from build123d import *

# Parameters (mm, degrees)
CYLINDER050_R           = 1.25
CYLINDER050_DEPTH       = 10
CYLINDER050_PITCH_ANGLE = 90
CYLINDER045_R           = 1.25
CYLINDER045_DEPTH       = 10
CYLINDER045_PITCH_ANGLE = 90
CYLINDER046_R           = 1.25
CYLINDER046_DEPTH       = 10
CYLINDER046_PITCH_ANGLE = 90
CYLINDER032_R           = 8.1
CYLINDER032_DEPTH       = 5
CYLINDER032_PITCH_ANGLE = 90
CYLINDER017_R           = 1.6
CYLINDER017_DEPTH       = 25
CYLINDER017_PITCH_ANGLE = 90
CYLINDER018_R           = 3.1
CYLINDER018_DEPTH       = 4
CYLINDER018_PITCH_ANGLE = 90
CYLINDER019_R           = 1.6
CYLINDER019_DEPTH       = 25
CYLINDER019_PITCH_ANGLE = 90
CYLINDER020_R           = 3.1
CYLINDER020_DEPTH       = 4
CYLINDER020_PITCH_ANGLE = 90
CYLINDER015_R           = 1.6
CYLINDER015_DEPTH       = 25
CYLINDER015_PITCH_ANGLE = 90
CYLINDER016_R           = 3.1
CYLINDER016_DEPTH       = 4
CYLINDER016_PITCH_ANGLE = 90
CYLINDER013_R           = 1.6
CYLINDER013_DEPTH       = 25
CYLINDER013_PITCH_ANGLE = 90
CYLINDER014_R           = 3.1
CYLINDER014_DEPTH       = 4
CYLINDER014_PITCH_ANGLE = 90
CYLINDER012_R           = 15.5
CYLINDER012_DEPTH       = 18
CYLINDER012_PITCH_ANGLE = 90
CYLINDER022_R           = 4
CYLINDER022_DEPTH       = 5
CYLINDER022_PITCH_ANGLE = 90
CYLINDER021_R           = 4
CYLINDER021_DEPTH       = 5
CYLINDER021_PITCH_ANGLE = 90
BOX007_W                = 33
BOX007_H                = 30
BOX007_DEPTH            = 40
CYLINDER003_R           = 17
CYLINDER003_DEPTH       = 19
CYLINDER003_PITCH_ANGLE = 90
BOX001_W                = 23
BOX001_H                = 30
BOX001_DEPTH            = 35
FILLET002_R             = 10
FILLET004_R             = 6
BOX_W                   = 32
BOX_H                   = 30
BOX_DEPTH               = 40
FILLET003_R             = 10
FILLET005_R             = 6


with BuildPart() as cylinder050:
    # Cylinder050 → Cylinder050 (new body)
    with BuildSketch(Plane.XY):
        Circle(CYLINDER050_R)
    extrude(amount=CYLINDER050_DEPTH)


with BuildPart() as cylinder050_1:
    # Cylinder050 pitch: moved
    add(cylinder050.part.rotate(Axis((0, 0, 0), (0, 1, 0)), CYLINDER050_PITCH_ANGLE))


with BuildPart() as cylinder050_2:
    # Cylinder050 placement: moved
    add(cylinder050_1.part.moved(Location((48, 15, 30))))


with BuildPart() as cylinder045:
    # Cylinder045 → Cylinder045 (new body)
    with BuildSketch(Plane.XY):
        Circle(CYLINDER045_R)
    extrude(amount=CYLINDER045_DEPTH)


with BuildPart() as cylinder045_1:
    # Cylinder045 pitch: moved
    add(cylinder045.part.rotate(Axis((0, 0, 0), (0, 1, 0)), CYLINDER045_PITCH_ANGLE))


with BuildPart() as cylinder045_2:
    # Cylinder045 placement: moved
    add(cylinder045_1.part.moved(Location((47, 7, 12))))


with BuildPart() as fusion023:
    # Cylinder046 → Cylinder046 (new body)
    with BuildSketch(Plane.XY):
        Circle(CYLINDER046_R)
    extrude(amount=CYLINDER046_DEPTH)


with BuildPart() as fusion023_1:
    # Cylinder046 pitch: moved
    add(fusion023.part.rotate(Axis((0, 0, 0), (0, 1, 0)), CYLINDER046_PITCH_ANGLE))


with BuildPart() as fusion023_2:
    # Cylinder046 placement: moved
    add(fusion023_1.part.moved(Location((46, 23, 12))))

    # Fusion023: union Cylinder045
    add(cylinder045_2.part)


with BuildPart() as cylinder032:
    # Cylinder032 → Cylinder032 (new body)
    with BuildSketch(Plane.XY):
        Circle(CYLINDER032_R)
    extrude(amount=CYLINDER032_DEPTH)


with BuildPart() as cylinder032_1:
    # Cylinder032 pitch: moved
    add(cylinder032.part.rotate(Axis((0, 0, 0), (0, 1, 0)), CYLINDER032_PITCH_ANGLE))


with BuildPart() as cylinder032_2:
    # Cylinder032 placement: moved
    add(cylinder032_1.part.moved(Location((51, 15, 19))))


with BuildPart() as cylinder017:
    # Cylinder017 → Cylinder017 (new body)
    with BuildSketch(Plane.XY):
        Circle(CYLINDER017_R)
    extrude(amount=CYLINDER017_DEPTH)


with BuildPart() as cylinder017_1:
    # Cylinder017 pitch: moved
    add(cylinder017.part.rotate(Axis((0, 0, 0), (0, 1, 0)), CYLINDER017_PITCH_ANGLE))


with BuildPart() as cylinder017_2:
    # Cylinder017 placement: moved
    add(cylinder017_1.part.moved(Location((30, 0, 19))))


with BuildPart() as fusion010:
    # Cylinder018 → Cylinder018 (new body)
    with BuildSketch(Plane.XY):
        Circle(CYLINDER018_R)
    extrude(amount=CYLINDER018_DEPTH)


with BuildPart() as fusion010_1:
    # Cylinder018 pitch: moved
    add(fusion010.part.rotate(Axis((0, 0, 0), (0, 1, 0)), CYLINDER018_PITCH_ANGLE))


with BuildPart() as fusion010_2:
    # Cylinder018 placement: moved
    add(fusion010_1.part.moved(Location((51, 0, 19))))

    # Fusion010: union Cylinder017
    add(cylinder017_2.part)


with BuildPart() as fusion010_3:
    # Fusion010 placement: moved
    add(fusion010_2.part.moved(Location((0, 25, 17))))


with BuildPart() as cylinder019:
    # Cylinder019 → Cylinder019 (new body)
    with BuildSketch(Plane.XY):
        Circle(CYLINDER019_R)
    extrude(amount=CYLINDER019_DEPTH)


with BuildPart() as cylinder019_1:
    # Cylinder019 pitch: moved
    add(cylinder019.part.rotate(Axis((0, 0, 0), (0, 1, 0)), CYLINDER019_PITCH_ANGLE))


with BuildPart() as cylinder019_2:
    # Cylinder019 placement: moved
    add(cylinder019_1.part.moved(Location((30, 0, 19))))


with BuildPart() as fusion011:
    # Cylinder020 → Cylinder020 (new body)
    with BuildSketch(Plane.XY):
        Circle(CYLINDER020_R)
    extrude(amount=CYLINDER020_DEPTH)


with BuildPart() as fusion011_1:
    # Cylinder020 pitch: moved
    add(fusion011.part.rotate(Axis((0, 0, 0), (0, 1, 0)), CYLINDER020_PITCH_ANGLE))


with BuildPart() as fusion011_2:
    # Cylinder020 placement: moved
    add(fusion011_1.part.moved(Location((51, 0, 19))))

    # Fusion011: union Cylinder019
    add(cylinder019_2.part)


with BuildPart() as fusion011_3:
    # Fusion011 placement: moved
    add(fusion011_2.part.moved(Location((0, 26, -14))))


with BuildPart() as cylinder015:
    # Cylinder015 → Cylinder015 (new body)
    with BuildSketch(Plane.XY):
        Circle(CYLINDER015_R)
    extrude(amount=CYLINDER015_DEPTH)


with BuildPart() as cylinder015_1:
    # Cylinder015 pitch: moved
    add(cylinder015.part.rotate(Axis((0, 0, 0), (0, 1, 0)), CYLINDER015_PITCH_ANGLE))


with BuildPart() as cylinder015_2:
    # Cylinder015 placement: moved
    add(cylinder015_1.part.moved(Location((30, 0, 19))))


with BuildPart() as fusion009:
    # Cylinder016 → Cylinder016 (new body)
    with BuildSketch(Plane.XY):
        Circle(CYLINDER016_R)
    extrude(amount=CYLINDER016_DEPTH)


with BuildPart() as fusion009_1:
    # Cylinder016 pitch: moved
    add(fusion009.part.rotate(Axis((0, 0, 0), (0, 1, 0)), CYLINDER016_PITCH_ANGLE))


with BuildPart() as fusion009_2:
    # Cylinder016 placement: moved
    add(fusion009_1.part.moved(Location((51, 0, 19))))

    # Fusion009: union Cylinder015
    add(cylinder015_2.part)


with BuildPart() as fusion009_3:
    # Fusion009 placement: moved
    add(fusion009_2.part.moved(Location((0, 5, 17))))


with BuildPart() as cylinder013:
    # Cylinder013 → Cylinder013 (new body)
    with BuildSketch(Plane.XY):
        Circle(CYLINDER013_R)
    extrude(amount=CYLINDER013_DEPTH)


with BuildPart() as cylinder013_1:
    # Cylinder013 pitch: moved
    add(cylinder013.part.rotate(Axis((0, 0, 0), (0, 1, 0)), CYLINDER013_PITCH_ANGLE))


with BuildPart() as cylinder013_2:
    # Cylinder013 placement: moved
    add(cylinder013_1.part.moved(Location((30, 0, 19))))


with BuildPart() as fusion013:
    # Cylinder014 → Cylinder014 (new body)
    with BuildSketch(Plane.XY):
        Circle(CYLINDER014_R)
    extrude(amount=CYLINDER014_DEPTH)


with BuildPart() as fusion013_1:
    # Cylinder014 pitch: moved
    add(fusion013.part.rotate(Axis((0, 0, 0), (0, 1, 0)), CYLINDER014_PITCH_ANGLE))


with BuildPart() as fusion013_2:
    # Cylinder014 placement: moved
    add(fusion013_1.part.moved(Location((51, 0, 19))))

    # Fusion008: union Cylinder013
    add(cylinder013_2.part)


with BuildPart() as fusion013_3:
    # Fusion008 placement: moved
    add(fusion013_2.part.moved(Location((0, 4, -14))))

    # Fusion013: union Fusion010, Fusion011, Fusion009
    add(fusion010_3.part)
    add(fusion011_3.part)
    add(fusion009_3.part)


with BuildPart() as fusion013_4:
    # Fusion013 placement: moved
    add(fusion013_3.part.moved(Location((1, 0, 0))))


with BuildPart() as cylinder012:
    # Cylinder012 → Cylinder012 (new body)
    with BuildSketch(Plane.XY):
        Circle(CYLINDER012_R)
    extrude(amount=CYLINDER012_DEPTH)


with BuildPart() as cylinder012_1:
    # Cylinder012 pitch: moved
    add(cylinder012.part.rotate(Axis((0, 0, 0), (0, 1, 0)), CYLINDER012_PITCH_ANGLE))


with BuildPart() as cylinder012_2:
    # Cylinder012 placement: moved
    add(cylinder012_1.part.moved(Location((33, 15, 19))))


with BuildPart() as cylinder022:
    # Cylinder022 → Cylinder022 (new body)
    with BuildSketch(Plane.XY):
        Circle(CYLINDER022_R)
    extrude(amount=CYLINDER022_DEPTH)


with BuildPart() as cylinder022_1:
    # Cylinder022 pitch: moved
    add(cylinder022.part.rotate(Axis((0, 0, 0), (0, 1, 0)), CYLINDER022_PITCH_ANGLE))


with BuildPart() as cylinder022_2:
    # Cylinder022 placement: moved
    add(cylinder022_1.part.moved(Location((50, 26, 5))))


with BuildPart() as cylinder021:
    # Cylinder021 → Cylinder021 (new body)
    with BuildSketch(Plane.XY):
        Circle(CYLINDER021_R)
    extrude(amount=CYLINDER021_DEPTH)


with BuildPart() as cylinder021_1:
    # Cylinder021 pitch: moved
    add(cylinder021.part.rotate(Axis((0, 0, 0), (0, 1, 0)), CYLINDER021_PITCH_ANGLE))


with BuildPart() as cylinder021_2:
    # Cylinder021 placement: moved
    add(cylinder021_1.part.moved(Location((50, 4, 5))))


with BuildPart() as box007:
    # Box007 → Box007 (new body)
    with BuildSketch(Plane.XY):
        with Locations((16.5, 15)):
            Rectangle(BOX007_W, BOX007_H)
    extrude(amount=BOX007_DEPTH)


with BuildPart() as cylinder003:
    # Cylinder003 → Cylinder003 (new body)
    with BuildSketch(Plane.XY):
        Circle(CYLINDER003_R)
    extrude(amount=CYLINDER003_DEPTH)


with BuildPart() as cylinder003_1:
    # Cylinder003 pitch: moved
    add(cylinder003.part.rotate(Axis((0, 0, 0), (0, 1, 0)), CYLINDER003_PITCH_ANGLE))


with BuildPart() as cylinder003_2:
    # Cylinder003 placement: moved
    add(cylinder003_1.part.moved(Location((33, 15, 19))))


with BuildPart() as fillet004:
    # Box001 → Box001 (new body)
    with BuildSketch(Plane.XY.offset(5)):
        with Locations((11.5, 15)):
            Rectangle(BOX001_W, BOX001_H)
    extrude(amount=BOX001_DEPTH)

    # Fillet002
    fillet002_edges = [fillet004.edges().sort_by_distance(p)[0] for p in [
        (11.5, 0, 5),
        (11.5, 30, 5),
    ]]
    fillet(fillet002_edges, radius=FILLET002_R)

    # Fillet004
    fillet004_edges = [fillet004.edges().sort_by_distance(p)[0] for p in [
        (11.5, 0, 40),
        (11.5, 30, 40),
    ]]
    fillet(fillet004_edges, radius=FILLET004_R)


with BuildPart() as rear_part:
    # Box → Box (new body)
    with BuildSketch(Plane(origin=(23, 0, 0), x_dir=(1, 0, 0), z_dir=(0, 0, 1))):
        with Locations((16, 15)):
            Rectangle(BOX_W, BOX_H)
    extrude(amount=BOX_DEPTH)

    # Fillet003
    fillet003_edges = [rear_part.edges().sort_by_distance(p)[0] for p in [
        (39, 0, 0),
        (39, 30, 0),
    ]]
    fillet(fillet003_edges, radius=FILLET003_R)

    # Fillet005
    fillet005_edges = [rear_part.edges().sort_by_distance(p)[0] for p in [
        (39, 0, 40),
        (39, 30, 40),
    ]]
    fillet(fillet005_edges, radius=FILLET005_R)

    # Fusion004: union Fillet004
    add(fillet004.part)

    # Fusion006: union Cylinder003
    add(cylinder003_2.part)

    # Cut005: cut Box007
    add(box007.part, mode=Mode.SUBTRACT)

    # Fusion014: union Cylinder022, Cylinder021
    add(cylinder022_2.part)
    add(cylinder021_2.part)

    # Cut007: cut Cylinder012
    add(cylinder012_2.part, mode=Mode.SUBTRACT)

    # Cut008: cut Fusion013
    add(fusion013_4.part, mode=Mode.SUBTRACT)

    # Cut011: cut Cylinder032
    add(cylinder032_2.part, mode=Mode.SUBTRACT)

    # Cut015: cut Fusion023
    add(fusion023_2.part, mode=Mode.SUBTRACT)

    # Cut018: cut Cylinder050
    add(cylinder050_2.part, mode=Mode.SUBTRACT)


solid = rear_part.part
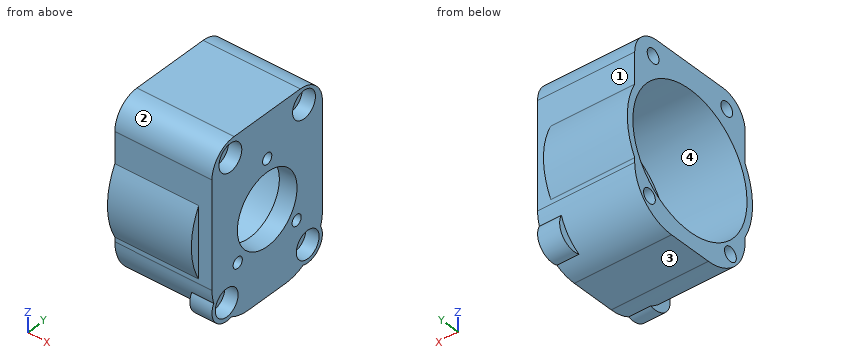
Model file for the job. Use its own axes, mm. Face numbers are marked on the shaded views. Coordinates: 2 decimals unless noted, no trailing zeros. Write each loop counter-clockwise with the first axis right and the second up, starting at its lowest first coordinate (ties: lowest second). Pieces come first, ordered by that corner, then holes. Notation, with made-up numbers: (-13.75, 46) - (3.25, 46) arc R29 cw to (3.25, 82) - close; hole circle Ø11 at (36, -1). An arc over 180 degrees is marked (long way). Write each question's results on one line, items separated by ' | '. Start each with the question number.
1) Mould opens along Z. For the marked faces 1, 2, 3 and 4 say: pulls with the +Z half, pulls with the -Z half, needs draft (parallel to the pull), parting line crosses it, or undercut.
2) Probe line 1 along Z through (x, y) = (52.2, 15); line 2 along Y through (x, z) = (34.5, 19); line 3 along Z through (x, y) = (54.1, 26). List the from-to ranges inside material, lowest first. Write a range as from..to.
3) Cut at D-D (z = 12). Write the cut outline in (x, y), then the cut area to 3 significant figures.
4) Flat gauge pins, fed straight in: P1, Ø1.5, axis at x = 46, y = 5, coming from the +Z side; P2, Ø3.5, axis at y = 25, z = 36, coming from the +X side; P3, Ø2, axis at x = 52.5, y = 8, coming from the -Z side. Where does each tip first touch, or does it go through?
5) Cut at B-B (z = 5). Write the cut outline in (x, y), then the cut area to 3 significant figures.
6) Cut at C-C (x = 42.25). Write the cut outline in (y, z).
7) Cut at A-A (y = 15). Write the cut outline in (x, z).
Returned:
1) face 1: needs draft | face 2: pulls with the +Z half | face 3: pulls with the -Z half | face 4: undercut
2) line 1: 0..10.9, 27.1..28.75, 31.25..40 | line 2: -2..-0.5, 30.5..32 | line 3: 1..1.9, 8.1..33.07, 38.93..39.66
3) outline: (33, -0.49) - (52, -0.49) - (52, 0) - (55, 0) - (55, 5.75) - (51, 5.75) - (51, 1.17) - (33, 1.17) - close; (33, 28.83) - (51, 28.83) - (51, 24.25) - (55, 24.25) - (55, 30) - (52, 30) - (52, 30.49) - (33, 30.49) - close; (51, 8.25) - (55, 8.25) - (55, 10.92) - (51, 10.92) - close; (51, 19.08) - (55, 19.08) - (55, 21.75) - (51, 21.75) - close | area: 128 mm^2
4) P1: z = 39.99 | P2: x = 52 | P3: z = 0.05
5) outline: (33, 1.34) - (50, 1.34) - (50, 0) - (55, 0) - (55, 0.9) - (52, 0.9) - (52, 2.4) - (33, 2.4) - close; (33, 5.6) - (52, 5.6) - (52, 7.1) - (55, 7.1) - (55, 22.9) - (52, 22.9) - (52, 24.4) - (33, 24.4) - (33, 21.65) - (51, 21.65) - (51, 8.35) - (33, 8.35) - close; (33, 27.6) - (52, 27.6) - (52, 29.1) - (55, 29.1) - (55, 30) - (50, 30) - (50, 28.66) - (33, 28.66) - close | area: 216 mm^2
6) outline: (0, 10) arc R10 ccw to (10, 0) - (20, 0) arc R10 ccw to (30, 10) - (30, 11) arc R17 ccw to (30, 27) - (30, 34) arc R6 ccw to (24, 40) - (6, 40) arc R6 ccw to (0, 34) - (0, 27) arc R17 ccw to (0, 11) - close; hole circle Ø31 at (15, 19); hole circle Ø3.2 at (4, 5); hole circle Ø3.2 at (5, 36); hole circle Ø3.2 at (25, 36); hole circle Ø3.2 at (26, 5)
7) outline: (33, 0) - (55, 0) - (55, 10.9) - (51, 10.9) - (51, 3.5) - (33, 3.5) - close; (33, 34.5) - (51, 34.5) - (51, 31.25) - (55, 31.25) - (55, 40) - (33, 40) - close; (51, 27.1) - (55, 27.1) - (55, 28.75) - (51, 28.75) - close
